For this review, take the finished solid that the model builds, in its own axes (mm). Face numbers are marked on the shaded views. A direction names the side the tool comes from. Give positions to 0.01 mm unless a question says otherwise; leave off trailing zeros. Order: outer loops, then holes, each group sorted by start corner. A loop starts at its lowest first (then second) coordinate and runs counter-clockwise, first axis right, second up. Notation, with made-up numbers: (64.25, 68.5) - (74.25, 68.5) arc R5 ccw to (74.25, 74.5) - close; hole circle Ø5 at (-4, -7.5). An arc over 180 degrees is marked (long way). Use a Markdown table: item, result. Add a question column.
1) Wall thickness on L1, parallel to X at y = 5.15, z = -10; L2, parallel to X at y = 8, z = -45; L3, parallel to X at y = 4, z = -34: over which ranges is each line inside the solid? List them lowest first.
2) We need section C-C on y = 2.75. Give the number of separate pieces and of enclosed holes in the cut face, then the cut area to 3 significant figures.
3) Machinability: for the marked faces 5 and 6, which of the approach directions +Z, -Z, +X, -X, +Y, -Y give a long, thin tool a straight path to every point of the face, cutting with its end or side? Answer none if there is none.
4) Mouldability with a two-part tool opening along Z and no side actions: class the marked faces 1, 2, 3 and 4 as released by +Z, released by -Z, zero draft, split by the parting line, or undercut.
5) We need section D-D on x = 21.4. Write out the cut boundary in (y, z).
6) We need section B-B on z = -35. Write out the cut boundary in (x, y), then the cut area to 3 significant figures.
7) Clearance check with a flat-ended pin moving along its axis: P1, Ø3, axis at x = 70, z = -4.8, coming from the +Y side. State where the tip first meets the part, or that it passes through.
8) We need section A-A on x = 37. Write out the cut boundary in (y, z), then the cut area to 3 significant figures.
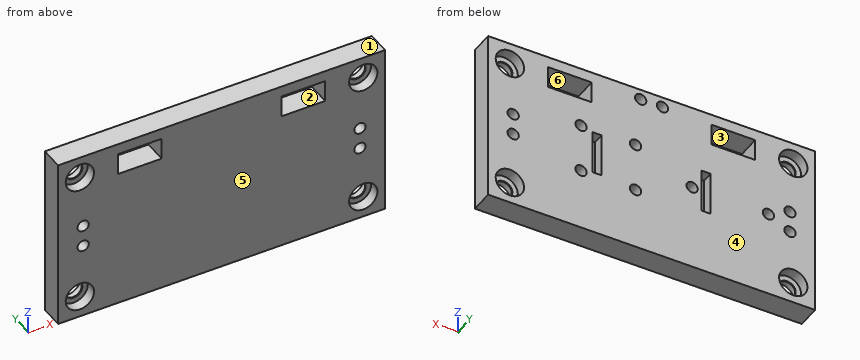
```python
from build123d import *

# Parameters (mm, degrees)
SKETCH1_W            = 150
SKETCH1_H            = 80
BOSS_EXTRUDE1_DEPTH  = 10.5
SKETCH10_R           = 6.5
CUT_EXTRUDE8_DEPTH   = 5
WIREHOLES_REACH      = 172.324
SKETCH3_W            = 20
SKETCH3_H            = 10
SKETCH6_R            = 2.6
F_4AACUT_DEPTH       = 5.2
SKETCH7_R            = 2.6
F_2AACUT_DEPTH       = 5.2
SKETCH5_W            = 4.2
SKETCH5_H            = 20.2
ARDUINOMEGACUT_DEPTH = 5.2
SKETCH8_R            = 2.6
MPUCUT_DEPTH         = 5.2
CUT_EXTRUDE7_REACH   = 172.324
SKETCH9_R            = 2.6
SKETCH11_R           = 4
CUT_EXTRUDE9_DEPTH   = 0.5


with BuildPart() as part:
    # Sketch1 → Boss-Extrude1 (new body)
    with BuildSketch(Plane(origin=(0, 0, 0), x_dir=(1, 0, 0), z_dir=(0, 1, 0))):
        with Locations((75, 40)):
            Rectangle(SKETCH1_W, SKETCH1_H)
    extrude(amount=BOSS_EXTRUDE1_DEPTH)

    # Sketch10 → Cut-Extrude8 (cut)
    with BuildSketch(Plane(origin=(0, 10.5, 0), x_dir=(1, 0, 0), z_dir=(0, 1, 0))):
        with Locations(Location((10, 10, 0), (0, 0, 270))):
            Circle(SKETCH10_R)
        with Locations(Location((140, 10, 0), (0, 0, 270))):
            Circle(SKETCH10_R)
        with Locations(Location((10, 70, 0), (0, 0, 270))):
            Circle(SKETCH10_R)
        with Locations(Location((140, 70, 0), (0, 0, 270))):
            Circle(SKETCH10_R)
    cut_extrude8 = extrude(amount=-CUT_EXTRUDE8_DEPTH, mode=Mode.SUBTRACT)

    # Mirror1: Cut-Extrude8 across plane
    add(cut_extrude8.mirror(Plane.ZX.offset(5.25)), mode=Mode.SUBTRACT)

    # Sketch3 → WireHoles (cut, up to next)
    with BuildSketch(Plane(origin=(0, 10.5, 0), x_dir=(1, 0, 0), z_dir=(0, 1, 0)), mode=Mode.PRIVATE) as wireholes_sk1:
        with Locations((37.5, 10)):
            Rectangle(SKETCH3_W, SKETCH3_H)
    wireholes_tool1 = extrude(wireholes_sk1.sketch, amount=-WIREHOLES_REACH, mode=Mode.PRIVATE) & part.part
    # Sketch3 → WireHoles (cut, up to next)
    with BuildSketch(Plane(origin=(0, 10.5, 0), x_dir=(1, 0, 0), z_dir=(0, 1, 0)), mode=Mode.PRIVATE) as wireholes_sk2:
        with Locations((112.5, 10)):
            Rectangle(SKETCH3_W, SKETCH3_H)
    wireholes_tool2 = extrude(wireholes_sk2.sketch, amount=-WIREHOLES_REACH, mode=Mode.PRIVATE) & part.part
    add(wireholes_tool1.solids().sort_by_distance((37.5, 10.5, -10))[0], mode=Mode.SUBTRACT)
    add(wireholes_tool2.solids().sort_by_distance((112.5, 10.5, -10))[0], mode=Mode.SUBTRACT)

    # Sketch6 → 4AACut (cut)
    with BuildSketch(Plane(origin=(0, 10.5, 0), x_dir=(1, 0, 0), z_dir=(0, 1, 0))):
        with Locations(Location((21.4, 40, 0), (0, 0, 270))):
            Circle(SKETCH6_R)
        with Locations(Location((56.4, 40, 0), (0, 0, 90))):
            Circle(SKETCH6_R)
    extrude(amount=-F_4AACUT_DEPTH, mode=Mode.SUBTRACT)

    # Sketch7 → 2AACut (cut)
    with BuildSketch(Plane(origin=(0, 10.5, 0), x_dir=(1, 0, 0), z_dir=(0, 1, 0))):
        with Locations(Location((82.35, 51.35, 0), (0, 0, 270))):
            Circle(SKETCH7_R)
        with Locations(Location((107.35, 51.35, 0), (0, 0, 90))):
            Circle(SKETCH7_R)
        with Locations(Location((82.35, 28.65, 0), (0, 0, 90))):
            Circle(SKETCH7_R)
        with Locations(Location((107.35, 28.65, 0), (0, 0, 270))):
            Circle(SKETCH7_R)
    extrude(amount=-F_2AACUT_DEPTH, mode=Mode.SUBTRACT)

    # Sketch5 → ArduinoMegaCut (cut)
    with BuildSketch(Plane(origin=(0, 10.5, 0), x_dir=(1, 0, 0), z_dir=(0, 1, 0))):
        with Locations((50, 40)):
            Rectangle(SKETCH5_W, SKETCH5_H)
        with Locations((100, 40)):
            Rectangle(SKETCH5_W, SKETCH5_H)
    extrude(amount=-ARDUINOMEGACUT_DEPTH, mode=Mode.SUBTRACT)

    # Sketch8 → MPUCut (cut)
    with BuildSketch(Plane(origin=(0, 10.5, 0), x_dir=(1, 0, 0), z_dir=(0, 1, 0))):
        with Locations(Location((70, 4.8, 0), (0, 0, 270))):
            Circle(SKETCH8_R)
        with Locations(Location((80, 4.8, 0), (0, 0, 90))):
            Circle(SKETCH8_R)
    extrude(amount=-MPUCUT_DEPTH, mode=Mode.SUBTRACT)

    # Sketch9 → Cut-Extrude7 (cut, up to next)
    with BuildSketch(Plane(origin=(0, 10.5, 0), x_dir=(1, 0, 0), z_dir=(0, 1, 0)), mode=Mode.PRIVATE) as cut_extrude7_sk1:
        with Locations(Location((138.5, 45, 0), (0, 0, 270))):
            Circle(SKETCH9_R)
    cut_extrude7_tool1 = extrude(cut_extrude7_sk1.sketch, amount=-CUT_EXTRUDE7_REACH, mode=Mode.PRIVATE) & part.part
    # Sketch9 → Cut-Extrude7 (cut, up to next)
    with BuildSketch(Plane(origin=(0, 10.5, 0), x_dir=(1, 0, 0), z_dir=(0, 1, 0)), mode=Mode.PRIVATE) as cut_extrude7_sk2:
        with Locations(Location((138.5, 35, 0), (0, 0, 270))):
            Circle(SKETCH9_R)
    cut_extrude7_tool2 = extrude(cut_extrude7_sk2.sketch, amount=-CUT_EXTRUDE7_REACH, mode=Mode.PRIVATE) & part.part
    # Sketch9 → Cut-Extrude7 (cut, up to next)
    with BuildSketch(Plane(origin=(0, 10.5, 0), x_dir=(1, 0, 0), z_dir=(0, 1, 0)), mode=Mode.PRIVATE) as cut_extrude7_sk3:
        with Locations(Location((11.5, 45, 0), (0, 0, 270))):
            Circle(SKETCH9_R)
    cut_extrude7_tool3 = extrude(cut_extrude7_sk3.sketch, amount=-CUT_EXTRUDE7_REACH, mode=Mode.PRIVATE) & part.part
    # Sketch9 → Cut-Extrude7 (cut, up to next)
    with BuildSketch(Plane(origin=(0, 10.5, 0), x_dir=(1, 0, 0), z_dir=(0, 1, 0)), mode=Mode.PRIVATE) as cut_extrude7_sk4:
        with Locations(Location((11.5, 35, 0), (0, 0, 270))):
            Circle(SKETCH9_R)
    cut_extrude7_tool4 = extrude(cut_extrude7_sk4.sketch, amount=-CUT_EXTRUDE7_REACH, mode=Mode.PRIVATE) & part.part
    add(cut_extrude7_tool1.solids().sort_by_distance((138.5, 10.5, -45))[0], mode=Mode.SUBTRACT)
    add(cut_extrude7_tool2.solids().sort_by_distance((138.5, 10.5, -35))[0], mode=Mode.SUBTRACT)
    add(cut_extrude7_tool3.solids().sort_by_distance((11.5, 10.5, -45))[0], mode=Mode.SUBTRACT)
    add(cut_extrude7_tool4.solids().sort_by_distance((11.5, 10.5, -35))[0], mode=Mode.SUBTRACT)

    # Sketch11 → Cut-Extrude9 (cut)
    with BuildSketch(Plane(origin=(0, 5.5, 0), x_dir=(1, 0, 0), z_dir=(0, 1, 0))):
        with Locations(Location((10, 10, 0), (0, 0, 270))):
            Circle(SKETCH11_R)
        with Locations(Location((10, 70, 0), (0, 0, 90))):
            Circle(SKETCH11_R)
        with Locations(Location((140, 70, 0), (0, 0, 270))):
            Circle(SKETCH11_R)
        with Locations(Location((140, 10, 0), (0, 0, 90))):
            Circle(SKETCH11_R)
    extrude(amount=-CUT_EXTRUDE9_DEPTH, mode=Mode.SUBTRACT)


solid = part.part
```
Checked values:
| question | item | result |
|---|---|---|
| 1 | L1 | 0 to 6, 14 to 27.5, 47.5 to 102.5, 122.5 to 136, 144 to 150 |
| 1 | L2 | 0 to 8.9, 14.1 to 47.9, 52.1 to 97.9, 102.1 to 135.9, 141.1 to 150 |
| 1 | L3 | 0 to 9.1, 13.9 to 136.1, 140.9 to 150 |
| 2 | separate pieces | 1 |
| 2 | enclosed holes | 10 |
| 2 | area | 11,000 mm² |
| 3 | face 5 | +Z, -Z, +X, -X, -Y |
| 3 | face 6 | +Y, -Y |
| 4 | face 1 | released by +Z |
| 4 | face 2 | undercut |
| 4 | face 3 | undercut |
| 4 | face 4 | zero draft |
| 5 | outline | (0, -80) - (10.5, -80) - (10.5, -42.6) - (5.3, -42.6) - (5.3, -37.4) - (10.5, -37.4) - (10.5, 0) - (0, 0) - close |
| 6 | outline | (0, 0) - (8.9, 0) - (8.9, 10.5) - (0, 10.5) - close; (14.1, 0) - (135.9, 0) - (135.9, 10.5) - (102.1, 10.5) - (102.1, 5.3) - (97.9, 5.3) - (97.9, 10.5) - (52.1, 10.5) - (52.1, 5.3) - (47.9, 5.3) - (47.9, 10.5) - (14.1, 10.5) - close; (141.1, 0) - (150, 0) - (150, 10.5) - (141.1, 10.5) - close |
| 6 | area | 1,420 mm² |
| 7 | P1 | y = 5.3 |
| 8 | outline | (0, -80) - (10.5, -80) - (10.5, -15) - (0, -15) - close; (0, -5) - (10.5, -5) - (10.5, 0) - (0, 0) - close |
| 8 | area | 735 mm² |
